Autodesk Inventor part; units mm, degrees
ref_plane "Start plane" through (0, 0, -7.8501) normal (0, 0, 1) x (1, 0, 0)
ref_plane "End plane" through (0, 0, 463.5299) normal (0, 0, 1) x (1, 0, 0)
ref_plane "Work Plane7" through (-113.0825, 0, 23.7264) normal (-0.2588, 0, -0.9659) x (-0.9659, 0, 0.2588)
ref_plane "Start plane" through (0, 0, -7.8501) normal (0, 0, 1) x (1, 0, 0)
ref_plane "End plane" through (0, 0, 463.5299) normal (0, 0, 1) x (1, 0, 0)
sketch "Sketch" plane through (0, 0, 0) normal (0, 0, 1) x (1, 0, 0)
  line L0 (4.7625, -6.35) -> (-4.7625, -6.35)
  line L1 (-4.7625, -6.35) -> (-4.7625, 6.35)
  line L2 (-4.7625, 6.35) -> (4.7625, 6.35)
  line L3 (4.7625, 6.35) -> (4.7625, -6.35)
  line L4 (-6, 0) -> (8, 0) construction
  line L5 (0, -30) -> (0, 40) construction
  line L6 (0, 54) -> (0, -44) construction
  line L7 (-9.2, 0) -> (13.2, 0) construction
  dimension "d0" = 12.7
  dimension "d1" = 9.525
  dimension "d4" = 4.7625
  dimension "d5" = 6.35
extrude "Body" add sketch "Sketch" along normal up to surface (471.38 mm away) from surface at -7.8501
sketch "Sketch3" plane through (0, 0, 0) normal (0, 0, 1) x (1, 0, 0)
  line L0 (0, 0) -> (10, 0)
ref_plane "Work Plane3" through (0, 0, 0) normal (0, -1, 0) x (1, 0, 0)
sketch "Sketch4" plane through (0, 0, 0) normal (0, -1, 0) x (1, 0, 0)
  line L0 (-2, -7.8501) -> (12, -7.8501)
  line L1 (-2, 463.5299) -> (12, 463.5299)
  dimension "d9" = 471.38
ref_plane "Work Plane7" through (-113.0825, 0, 23.7264) normal (-0.2588, 0, -0.9659) x (-0.9659, 0, 0.2588)
split "Split4" plane through (-113.0825, 0, 23.7264) removes the side toward (-0.2588, 0, -0.9659)
ref_plane "Work Plane8" through (41.265, -6.35, 599.759) normal (-0.9659, 0, 0.2588) x (0.2588, 0, 0.9659)
split "Split5" plane through (41.265, -6.35, 599.759) removes the side toward (-0.9659, 0, 0.2588)
equation "\"d0\" = G_W"
equation "\"d1\" = G_H"
equation "\"d4\" = 0.5 * d1"
equation "\"d5\" = 0.5 * d0"
equation "\"d2\" = G_L"
equation "\"G_W\" = 12.7"
equation "\"G_H\" = 9.525"
equation "\"G_L\" = d9"
equation "\"G_OFFSET_START\" = 7.85011"
equation "\"G_OFFSET_END\" = -6.76062"
equation "\"d6\" = -G_OFFSET_START"
equation "\"d7\" = G_OFFSET_END + B_L"
equation "\"B_L\" = 470.29055"
properties part number "AISC - 1/2x3/8 - 18.558" material "Steel, Alloy"
Here's how the part is built. I have some questions about the finished solid (model axes, mm). Give positions to 0.01 mm unless a question says otherwise; leave off trailing zeros. Write each loop counter-clockwise with the first axis right and the second up, starting at its lowest first coordinate (ties: lowest second). Pieces come first, ordered by that corner, then holes. Notation, with made-up numbers: (76, 82.5) -> (105, 82.5) arc R35 ccw to (105, 114.5) -> close; hole circle Ø7 at (11.25, -26). An arc over 180 degrees is marked (long way). Use one line per item in the form item = value.
1) If I drill on L1, parallel to X at y = -1.5, z = 430; L2, parallel to X at y = -5.5, z = 443, over which ranges is the centre line in solid material (lowest first)? Write a range as [from, to].
Verdict:
L1 = [-4.22, 4.76]
L2 = [-0.74, 4.76]
2) Suppose I cut it at A-A (y = -2.75). Please give me the cut outline in (x, z), and give its area (3 significant figures).
Verdict:
outline = (-4.76, -5.3) -> (4.76, -7.85) -> (4.76, 463.53) -> (-4.76, 427.98) -> close
area = 4,310 mm2
3) Suppose I cut it at B-B (x = -0.5). Please give me the cut outline in (y, z), and give its area (3 significant figures).
Verdict:
outline = (-6.35, -6.44) -> (6.35, -6.44) -> (6.35, 443.89) -> (-6.35, 443.89) -> close
area = 5,720 mm2
